```python
from build123d import *

# Parameters (mm, degrees)
BOSS_EXTRUDE1_DEPTH = 25
SKETCH2_W           = 15
SKETCH2_H           = 30
CUT_EXTRUDE1_DEPTH  = 30
SKETCH3_R           = 2.5
BOSS_EXTRUDE2_DEPTH = 10
BOSS_EXTRUDE3_REACH = 69.5
SKETCH5_R           = 2.5


with BuildPart() as part:
    # Sketch1 → Boss-Extrude1 (new body)
    with BuildSketch(Plane(origin=(0, 0, 0), x_dir=(1, 0, 0), z_dir=(0, 1, 0))):
        Polygon((-50, 20), (50, 20), (50, 0), (15, 0), (15, -45), (-15, -45), (-15, 0), (-50, 0), align=None)
    extrude(amount=BOSS_EXTRUDE1_DEPTH)

    # Sketch2 → Cut-Extrude1 (cut)
    with BuildSketch(Plane.XY.offset(45)):
        with Locations((0, 15)):
            Rectangle(SKETCH2_W, SKETCH2_H)
    extrude(amount=-CUT_EXTRUDE1_DEPTH, mode=Mode.SUBTRACT)

    # Sketch3 → Boss-Extrude2 (add)
    with BuildSketch(Plane(origin=(50, 0, 0), x_dir=(0, 0, -1), z_dir=(1, 0, 0))):
        with Locations((10, 10)):
            Circle(SKETCH3_R)
    boss_extrude2 = extrude(amount=BOSS_EXTRUDE2_DEPTH)

    # Mirror1: Boss-Extrude2 across plane
    add(boss_extrude2.mirror(Plane(origin=(0, 0, 0), x_dir=(0, 0, 1), z_dir=(1, 0, 0))))

    # Sketch5 → Boss-Extrude3 (add, up to next)
    with BuildSketch(Plane(origin=(-7.5, 0, 0), x_dir=(0, 0, -1), z_dir=(1, 0, 0)), mode=Mode.PRIVATE) as boss_extrude3_sk1:
        with Locations((-35, 10)):
            Circle(SKETCH5_R)
    boss_extrude3_tool1 = extrude(boss_extrude3_sk1.sketch, amount=BOSS_EXTRUDE3_REACH, mode=Mode.PRIVATE) - part.part
    add(boss_extrude3_tool1.solids().sort_by_distance((-7.5, 10, 35))[0])


solid = part.part
```
Can you work these out from the model? Positions are in its coordinate system, mm. A direction names the side the tool comes from. Coordinates: 2 decimals unless noted, no trailing zeros. Loops run counter-clockwise (first coordinate to the right, second up) from the corner with the lowest first, then second, coordinate; pieces in that order, holes last. Notation, with made-up numbers: M 20,-35.75 L 58,-35.75 A28 cw 58,-11.75 Z; hole C 4.5,57.5 d10. An arc over 180 degrees is marked long. Put each result on its own line as item: value. Start each with the question number.
(1) Will these pins go through, and if not, where does the flat tip stop? pin 1 Ø12 at (x, y) = (0, 16) entering from +Z; pin 2 Ø1 at (y, z) = (4, 22) entering from -X; pin 3 Ø3 at (x, y) = (19.5, 4.5) entering from +Z.
(2) We'd pull the mould along X, two halves only. Please class faces 1 (the face through (1, 0, -2)), 2 (the face through (-60, 10, -10)), 3 (the face through (7.5, 12, 30)): +X half, -X half, draft (parallel to the pull), parting line (faces both ways), or undercut.
(3) Imagine slicing it at B-B on y = 18.75. List the corners of the cut face in (x, z) for me.
(4) Imagine slicing it at D-D on z = -10. List the corners of the cut face in (x, y) for me.
(5) Imagine slicing it at C-C on y = 10. List the corners of the cut face in (x, z) for me.
(6) Which directions (+Z, -Z, +X, -X, +Y, -Y) give clear straight access to the entire face, cutting with the end or side of a thin tool? Please do faces 4 (the face through (-54.93, 7.56, -9.46)), 5 (the face through (-32, 12, 0)), 6 (the face through (-0.11, 9.04, 32.69)), 7 (the face through (54.93, 7.56, -9.46)), 8 (the face through (15, 12, 22)).
(7) I need wall thicknesses on probe 1 along X at (y, z) = (15.5, 33); probe 2 along X at (y, z) = (14.5, 14); probe 3 along Z at (x, y) = (34, 15). Which ranges of each line are inside material? Lowest first, please.
(8) Imagine slicing it at A-A on z = 39. List the corners of the cut face in (x, y) for me, and give its area (3 significant figures).
Worked answers:
1. pin 1: stops at z = 37.5
1. pin 2: stops at x = -15
1. pin 3: stops at z = 0
2. face 1: draft
2. face 2: -X half
2. face 3: undercut
3. outline: M -50,-20 L 50,-20 L 50,0 L 15,0 L 15,45 L 7.5,45 L 7.5,15 L -7.5,15 L -7.5,45 L -15,45 L -15,0 L -50,0 Z
4. outline: M -60,7.5 L -50,7.5 L -50,0 L 50,0 L 50,7.5 L 60,7.5 L 60,12.5 L 50,12.5 L 50,25 L -50,25 L -50,12.5 L -60,12.5 Z
5. outline: M -60,-12.5 L -50,-12.5 L -50,-20 L 50,-20 L 50,-12.5 L 60,-12.5 L 60,-7.5 L 50,-7.5 L 50,0 L 15,0 L 15,45 L 7.5,45 L 7.5,37.5 L -7.5,37.5 L -7.5,45 L -15,45 L -15,0 L -50,0 L -50,-7.5 L -60,-7.5 Z; hole M -7.5,15 L 7.5,15 L 7.5,32.5 L -7.5,32.5 Z
6. face 4: -X
6. face 5: +Z, -X, +Y, -Y
6. face 6: none
6. face 7: +X
6. face 8: +Z, +X, +Y, -Y
7. probe 1: x = -15 to -7.5, 7.5 to 15
7. probe 2: x = -15 to 15
7. probe 3: z = -20 to 0
8. outline: M -15,0 L -7.5,0 L -7.5,25 L -15,25 Z; M 7.5,0 L 15,0 L 15,25 L 7.5,25 Z
8. area: 375 mm2
